from build123d import *

# Parameters (mm, degrees)
F0_R     = 50
F1_DEPTH = 5
F2_R     = 5
F3_DEPTH = 25


with BuildPart() as f1:
    # F0 (on Top) → F1 (new body, symmetric)
    with BuildSketch(Plane.XY):
        Circle(F0_R)
    extrude(amount=F1_DEPTH, both=True)

    # F2 (on face) → F3 (join)
    with BuildSketch(Plane.XY.offset(5)):
        with Locations((0, 35)):
            Circle(F2_R)
        with Locations((30.310889, -17.5)):
            Circle(F2_R)
        with Locations((-30.310889, -17.5)):
            Circle(F2_R)
    extrude(amount=F3_DEPTH)


solid = f1.part
The listing builds one solid part. Answer for the finished solid, in the listing's coordinates (mm). A direction names the side the tool comes from. Round coordinates to 2 decimals unless told otherwise and drop trailing zeros. Order: outer loops, then holes, each group sorted by start corner. A loop starts at its lowest first (then second) coordinate and runs counter-clockwise, first axis right, second up. Notation, with made-up numbers: M 33,46 L 39,46 A21 ccw 39,67 Z; hole C 85,-37 d8. An arc over 180 degrees is marked long. Answer in a Markdown table with one row per item. Add a question column.
1) Which of the six approach directions +Z, -Z, +X, -X, +Y, -Y give full straight-line access (tool end or side, diameter ignored) to faces 4 (the face through (0, 35, 30)), 5 (the face through (26.34, -20.54, 17.32))?
2) Consider line 1 along Z through (x, y) = (37, 2); line 2 along X through (y, z) = (-14, 23.5); line 3 along X through (y, z) = (-15, 27.5). Determine where each line is inside the solid, lowest interval first. Write a range as from..to.
3) The part is cut by section C-C on y = 35. Determine the outline of the cut face in (x, z).
4) Determine the mould class of faces 1 (the face through (3, 39, 17)), 2 (the face through (-25.692, -19.415, 17.325)), 3 (the face through (-30, -17, 30)) for opening direction X: pulls with the +X half, pulls with the -X half, needs draft (parallel to the pull), parting line crosses it, or undercut.
5) The part is cut by section B-B on x = 0. Determine the outline of the cut face in (y, z), plus the area to 3 significant figures.
6) The part is cut by section D-D on y = -17.5. Determine the outline of the cut face in (x, z).
7) The part is cut by section A-A on z = 8.5. Determine the outline of the cut face in (x, y), plus the area to 3 significant figures.
8) Flat-ended cylindrical pins translate along their axes: pin 1 Ø1.5 at (x, z) = (-31.5, 2) entering from -Y; pin 2 Ø3 at (y, z) = (-37, 6) entering from -X; pin 3 Ø4 at (x, z) = (-7.5, 2.5) entering from +Y; pin 4 Ø3 at (x, z) = (-23, 25.5) entering from +Y. Find the tip coordinate at first contact, or state that the pin passes through.
Findings below:
| question | item | result |
|---|---|---|
| 1 | face 4 | +Z, +X, -X, +Y, -Y |
| 1 | face 5 | +Z |
| 2 | line 1 | z = -5..5 |
| 2 | line 2 | x = -33.88..-26.74, 26.74..33.88 |
| 2 | line 3 | x = -34.64..-25.98, 25.98..34.64 |
| 3 | outline | M -35.71,-5 L 35.71,-5 L 35.71,5 L 5,5 L 5,30 L -5,30 L -5,5 L -35.71,5 Z |
| 4 | face 1 | parting line crosses it |
| 4 | face 2 | undercut |
| 4 | face 3 | needs draft |
| 5 | outline | M -50,-5 L 50,-5 L 50,5 L 40,5 L 40,30 L 30,30 L 30,5 L -50,5 Z |
| 5 | area | 1,250 mm² |
| 6 | outline | M -46.84,-5 L 46.84,-5 L 46.84,5 L 35.31,5 L 35.31,30 L 25.31,30 L 25.31,5 L -25.31,5 L -25.31,30 L -35.31,30 L -35.31,5 L -46.84,5 Z |
| 7 | outline | C -30.31,-17.5 d10; C 0,35 d10; C 30.31,-17.5 d10 |
| 7 | area | 236 mm² |
| 8 | pin 1 | stops at y = -39.43 |
| 8 | pin 2 | stops at x = -34.82 |
| 8 | pin 3 | stops at y = 49.7 |
| 8 | pin 4 | passes through |
